Can you work these out from the model? Positions are in its coordinate system, mm. Face numbers are marked on the shaded views. A direction names the side the tool comes from. Round coordinates to 2 decimals unless told otherwise and drop trailing zeros. Loops run counter-clockwise (first coordinate to the right, second up) from the corner with the lowest first, then second, coordinate; pieces in that order, holes last. Notation, with made-up numbers: (12.5, 71.5) -> (69.5, 71.5) arc R16 cw to (69.5, 94.5) -> close; hole circle Ø5 at (9, 34). An arc over 180 degrees is marked (long way). Write item = value, one per line.
Autodesk Inventor part; units mm, degrees
ref_plane "YZ Plane" through (0, 0, 0) normal (1, 0, 0) x (0, 1, 0)
ref_plane "XZ Plane" through (0, 0, 0) normal (0, 1, 0) x (-1, 0, 0)
ref_plane "XY Plane" through (0, 0, 0) normal (0, 0, 1) x (1, 0, 0)
sketch "Sketch1" plane through (0, 0, 0) normal (1, 0, 0) x (0, 1, 0)
  line L0 (20, 9.9) -> (-20, 9.9)
  line L1 (-20, 9.9) -> (-20, -9.9)
  line L2 (-20, -9.9) -> (20, -9.9)
  line L3 (20, -9.9) -> (20, 9.9)
  point P0 (0, 0)
  point P1 (0, 9.9)
  point P2 (-20, 0)
  dimension "d0" = 19.8
  dimension "d1" = 40
extrude "Extrusion1" add sketch "Sketch1" along normal blind 1.8
sketch "Sketch2" plane through (1.8, 0, 0) normal (1, 0, 0) x (0, 0, -1)
  circle A0 centre (0, 14) radius 1.15
  line L0 (-9.9, -20) -> (9.9, -20)
  point P0 (0, 0)
  dimension "d4" = 2.3
  dimension "d5" = 34
extrude "Extrusion2" add sketch "Sketch2" along normal blind 10
thicken "Thicken1" operation add thickness 10 both sides no extend neighbours yes toward (0, 1, 0) faces at (0.6, -20, 3.3)
thicken "Thicken2" operation add thickness 5 both sides no extend neighbours yes toward (0, -1, 0) faces at (0.6, -10, 3.3)
thicken "Thicken3" operation add thickness 2 both sides no extend neighbours yes toward (0, 1, 0) faces at (0.6, -15, 3.3)
thicken "Thicken4" operation add thickness 4 both sides no extend neighbours yes toward (0, -1, 0) faces at (0.6, 20, -3.3)
thicken "Thicken5" operation add thickness 2 both sides no extend neighbours yes toward (0, -1, 0) faces at (0.6, -13, 3.3)
thicken "Thicken6" operation add thickness 5 both sides no extend neighbours yes toward (1, 0, 0) faces at (11.8, 13.5623, 0.2869)
properties part number "sample-transfer_slider"
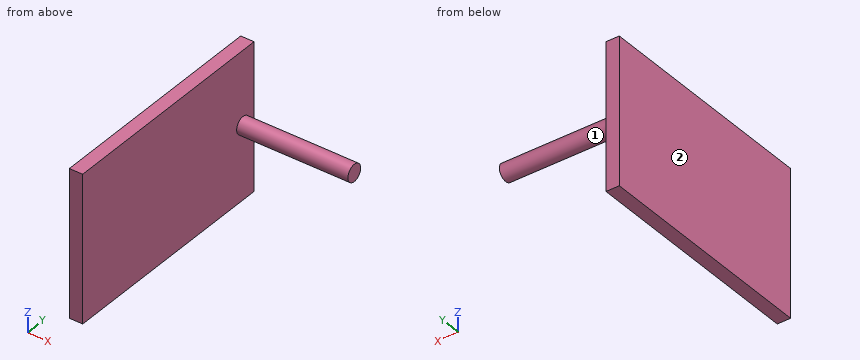
1. I need wall thicknesses on line 1 (X direction, y = 14.5, z = 8). Which ranges of the line are inside material? Lowest first, please. Write a range as [from, to].
Entries:
line_1 = [0, 1.8]
2. I'm going to push flat-ended pins straight in: pin 1 (5 mm diameter, centred on y = -8, z = 3.5, fed in from +X); pin 2 (10 mm diameter, centred on x = 10.5, y = 4.5, fed in from -Z). Where does each tip first touch, or does it pass through?
Entries:
pin_1 = 1.8
pin_2 = through
3. Suppose I cut it at B-B, the plane y = 14. List the corners of the cut face in (x, z) for me, and give its area (3 significant figures).
Entries:
outline = (0, -9.9) -> (1.8, -9.9) -> (1.8, -1.15) -> (16.8, -1.15) -> (16.8, 1.15) -> (1.8, 1.15) -> (1.8, 9.9) -> (0, 9.9) -> close
area = 70.1 mm²
4. Suppose I cut it at D-D, the plane y = 6.5. List the corners of the cut face in (x, z) for me, and give its area (3 significant figures).
Entries:
outline = (0, -9.9) -> (1.8, -9.9) -> (1.8, 9.9) -> (0, 9.9) -> close
area = 35.6 mm²
5. Suppose I cut it at C-C, the plane x = 12.25. List the corners of the cut face in (y, z) for me.
Entries:
outline = circle Ø2.3 at (14, 0)
6. Suppose I cut it at A-A, the plane z = 0. List the corners of the cut face in (x, y) for me.
Entries:
outline = (0, -15) -> (1.8, -15) -> (1.8, 12.85) -> (16.8, 12.85) -> (16.8, 15.15) -> (1.8, 15.15) -> (1.8, 16) -> (0, 16) -> close
7. For the marked faces 1 and 2, which set-ups out of +Z, -Z, +X, -X, +Y, -Y let a thin tool reach every point of the face, with its end or its side?
Entries:
face_1 = +X
face_2 = +Z, -Z, -X, +Y, -Y
